Build history of the part. All positions in model axes, mm. A direction names the side the tool comes from. Round coordinates to 2 decimals unless told otherwise and drop trailing zeros. Loops run counter-clockwise (first coordinate to the right, second up) from the corner with the lowest first, then second, coordinate; pieces in that order, holes last. Notation, with made-up numbers: (9, 86) - (67, 86) arc R10 ccw to (67, 96) - close; hole circle Ø3 at (88.25, 74.5). An arc over 180 degrees is marked (long way). Put each result on its own line as item: value. Start each with the question number.
from build123d import *

# Parameters (mm, degrees)
EXTRUDE_1_DEPTH          = 180
CUT_EXTRUDE_1_DEPTH      = 283.252103624
CUT_EXTRUDE_1_DEPTH_BACK = 283.252103624
SKETCH_13_R              = 70
SKETCH_13_R_2            = 2.5
CUT_EXTRUDE_2_DEPTH      = 50
SKETCH_14_R              = 2.5
CUT_EXTRUDE_3_DEPTH      = 6
SKETCH_15_R              = 30
SKETCH_15_R_2            = 2.25
CUT_EXTRUDE_4_DEPTH      = 6
FILLET_1_R               = 100
FILLET_2_R               = 80
FILLET_3_R               = 10


with BuildPart() as part:
    # 草图11 → 拉伸-薄壁1 (new body)
    with BuildSketch(Plane(origin=(0, 0, 0), x_dir=(0, 0, -1), z_dir=(1, 0, 0))):
        Polygon((-63.5, 0), (-63.5, 180), (-50, 200), (50, 200), (63.5, 180), (63.5, 0), (69.5, 0), (69.5, 181.835492011), (53.188957107, 206), (-53.188957107, 206), (-69.5, 181.835492011), (-69.5, 0), align=None)
    extrude(amount=EXTRUDE_1_DEPTH)

    # 草图12 → 切除-拉伸1 (cut, two sides: drawn at the far end of the back side and taken through both)
    with BuildSketch(Plane.XY.offset(-CUT_EXTRUDE_1_DEPTH_BACK)):
        Polygon((45, 206), (0, 106), (0, 206), align=None)
        Polygon((180, 106), (180, 206), (135, 206), align=None)
    extrude(amount=CUT_EXTRUDE_1_DEPTH + CUT_EXTRUDE_1_DEPTH_BACK, mode=Mode.SUBTRACT)

    # 草图13 → 切除-拉伸2 (cut)
    with BuildSketch(Plane(origin=(0, 0, -69.5), x_dir=(-1, 0, 0), z_dir=(0, 0, -1))):
        with Locations(Location((-90, 90, 0), (0, 0, 90))):
            Circle(SKETCH_13_R)
        with Locations(Location((-117.709167863, 166.379084286, 0), (0, 0, 90))):
            Circle(SKETCH_13_R_2)
        with Locations(Location((-142.291643378, 152.18638543, 0), (0, 0, 90))):
            Circle(SKETCH_13_R_2)
        with Locations(Location((-152.18638543, 142.291643378, 0), (0, 0, 90))):
            Circle(SKETCH_13_R_2)
        with Locations(Location((-166.379084286, 117.709167863, 0), (0, 0, 90))):
            Circle(SKETCH_13_R_2)
        with Locations(Location((-13.620915714, 117.709167863, 0), (0, 0, 90))):
            Circle(SKETCH_13_R_2)
        with Locations(Location((-27.81361457, 142.291643378, 0), (0, 0, 90))):
            Circle(SKETCH_13_R_2)
        with Locations(Location((-37.708356622, 152.18638543, 0), (0, 0, 90))):
            Circle(SKETCH_13_R_2)
        with Locations(Location((-62.290832137, 166.379084286, 0), (0, 0, 90))):
            Circle(SKETCH_13_R_2)
        with Locations(Location((-62.290832137, 13.620915714, 0), (0, 0, 90))):
            Circle(SKETCH_13_R_2)
        with Locations(Location((-37.708356622, 27.81361457, 0), (0, 0, 90))):
            Circle(SKETCH_13_R_2)
        with Locations(Location((-27.81361457, 37.708356622, 0), (0, 0, 90))):
            Circle(SKETCH_13_R_2)
        with Locations(Location((-13.620915714, 62.290832137, 0), (0, 0, 90))):
            Circle(SKETCH_13_R_2)
        with Locations(Location((-166.379084286, 62.290832137, 0), (0, 0, 90))):
            Circle(SKETCH_13_R_2)
        with Locations(Location((-152.18638543, 37.708356622, 0), (0, 0, 90))):
            Circle(SKETCH_13_R_2)
        with Locations(Location((-142.291643378, 27.81361457, 0), (0, 0, 90))):
            Circle(SKETCH_13_R_2)
        with Locations(Location((-117.709167863, 13.620915714, 0), (0, 0, 90))):
            Circle(SKETCH_13_R_2)
    extrude(amount=-CUT_EXTRUDE_2_DEPTH, mode=Mode.SUBTRACT)

    # 草图14 → 切除-拉伸3 (cut)
    with BuildSketch(Plane(origin=(0, 206, 0), x_dir=(1, 0, 0), z_dir=(0, 1, 0))):
        with Locations(Location((120, 5, 0), (0, 0, 270))):
            Circle(SKETCH_14_R)
        with Locations(Location((120, -25, 0), (0, 0, 90))):
            Circle(SKETCH_14_R)
        with Locations(Location((60, -25, 0), (0, 0, 270))):
            Circle(SKETCH_14_R)
        with Locations(Location((60, 5, 0), (0, 0, 90))):
            Circle(SKETCH_14_R)
    extrude(amount=-CUT_EXTRUDE_3_DEPTH, mode=Mode.SUBTRACT)

    # 草图15 → 切除-拉伸4 (cut)
    with BuildSketch(Plane.XY.offset(69.5)):
        with Locations((90, 90)):
            Circle(SKETCH_15_R)
        with Locations((90, 131.5)):
            Circle(SKETCH_15_R_2)
        with Locations((119.344931419, 119.344931419)):
            Circle(SKETCH_15_R_2)
        with Locations((131.5, 90)):
            Circle(SKETCH_15_R_2)
        with Locations((119.344931419, 60.655068581)):
            Circle(SKETCH_15_R_2)
        with Locations((90, 48.5)):
            Circle(SKETCH_15_R_2)
        with Locations((60.655068581, 60.655068581)):
            Circle(SKETCH_15_R_2)
        with Locations((48.5, 90)):
            Circle(SKETCH_15_R_2)
        with Locations((60.655068581, 119.344931419)):
            Circle(SKETCH_15_R_2)
    extrude(amount=-CUT_EXTRUDE_4_DEPTH, mode=Mode.SUBTRACT)

    # 圆角1
    fillet_1_edges = [part.edges().sort_by_distance(p)[0] for p in [
        (0, 106, 66.5),
        (180, 106, 66.5),
        (0, 106, -66.5),
        (180, 106, -66.5),
    ]]
    fillet(fillet_1_edges, radius=FILLET_1_R)

    # 圆角2
    fillet_2_edges = [part.edges().sort_by_distance(p)[0] for p in [
        (0, 0, -66.5),
        (0, 0, 66.5),
        (180, 0, -66.5),
        (180, 0, 66.5),
    ]]
    fillet(fillet_2_edges, radius=FILLET_2_R)

    # 圆角3
    fillet_3_edges = [part.edges().sort_by_distance(p)[0] for p in [
        (90, 181.835492011, 69.5),
        (90, 206, 53.188957107),
        (90, 206, -53.188957107),
        (90, 181.835492011, -69.5),
        (90, 180, -63.5),
        (90, 200, -50),
        (90, 200, 50),
        (90, 180, 63.5),
    ]]
    fillet(fillet_3_edges, radius=FILLET_3_R)


solid = part.part
1) Drill centre lines: line 1 (X direction, y = 202, z = -5); line 2 (Z direction, x = 22, y = 43.5); line 3 (Y direction, x = 90, z = 65.2). Where is each one in solid material? Low to high. Write a range as [from, to].
2) Slice it at A-A, the plane z = -5. Write the cut outline in (x, y), and give its area (3 significant figures).
3) Which spindle directions (+Z, -Z, +X, -X, +Y, -Y) get a long thin tool onto all of the face, cutting with end or side? Do faces 1 (the face through (26.3, 140.3, -66.5)), 2 (the face through (129, 91, 69.5)), 3 (the face through (90.696, 198.798, -49.439)). Say none if no direction does.
4) Pull direction X, two halves, no side cores. Call faces 4 (the face through (2.165, 105.233, 66.542)), 5 (the face through (13.731, 59.793, -66.542)), 6 (the face through (59.85, 13.08, -66.54)), 7 (the face through (89, 200, 1)): pulls with the +X half, pulls with the -X half, needs draft (parallel to the pull), parting line crosses it, or undercut.
5) Drop a flat-ended pin along its axis: pin 1 Ø4 at (x, y) = (166.38, 117.71) entering from -Z. Give the stop position or say it passes through.
6) Slice it at B-B, the plane z = -50.5. Write the cut outline in (x, y).
Taken from the geometry:
1. line 1: x = [43.2, 57.5], [62.5, 117.5], [122.5, 136.8]
1. line 2: z = [-69.5, -63.5], [63.5, 69.5]
1. line 3: y = [0, 46.25], [50.75, 60], [120, 129.25], [133.75, 188.21]
2. outline: (42.3, 200) - (57.5, 200) - (57.5, 206) - (45, 206) - close; (62.5, 200) - (117.5, 200) - (117.5, 206) - (62.5, 206) - close; (122.5, 200) - (137.7, 200) - (135, 206) - (122.5, 206) - close
2. area: 496 mm2
3. face 1: -Z
3. face 2: +Z, +X, -X, +Y, -Y
3. face 3: +X, -X, -Y
4. face 4: pulls with the -X half
4. face 5: undercut
4. face 6: undercut
4. face 7: needs draft
5. pin 1: stops at z = 63.5
6. outline: (41.46, 198.14) - (138.54, 198.14) - (135.16, 205.65) - (44.84, 205.65) - close
